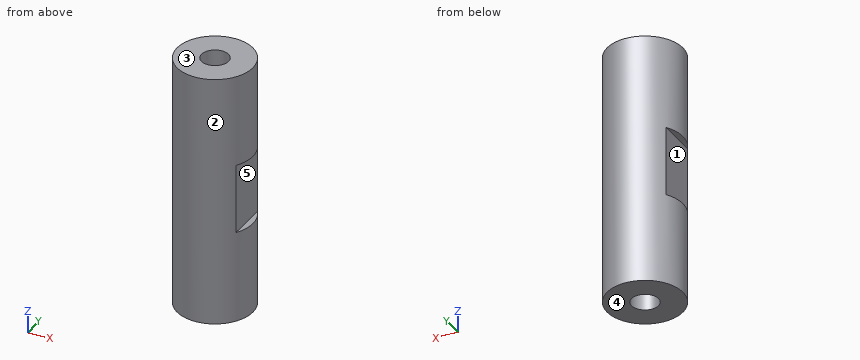
```python
from build123d import *

# Parameters (mm, degrees)
SKETCH_1_R               = 6
SKETCH_1_R_2             = 2.15
EXTRUDE_1_DEPTH          = 40
CUT_EXTRUDE_1_DEPTH      = 41.890096601
CUT_EXTRUDE_1_DEPTH_BACK = 41.890096601
SKETCH_2_W               = 1
SKETCH_2_H               = 11


with BuildPart() as part:
    # Эскиз1 → Бобышка-Вытянуть1 (new body)
    with BuildSketch(Plane.XY):
        Circle(SKETCH_1_R)
        Circle(SKETCH_1_R_2, mode=Mode.SUBTRACT)
    extrude(amount=EXTRUDE_1_DEPTH)

    # Эскиз2 → Вырез-Вытянуть1 (cut, two sides: drawn at the far end of the back side and taken through both)
    with BuildSketch(Plane(origin=(0, 0, 0), x_dir=(1, 0, 0), z_dir=(0, 1, 0)).offset(-CUT_EXTRUDE_1_DEPTH_BACK)):
        with Locations((-5.5, -20)):
            Rectangle(SKETCH_2_W, SKETCH_2_H)
        with Locations((5.5, -20)):
            Rectangle(SKETCH_2_W, SKETCH_2_H)
    extrude(amount=CUT_EXTRUDE_1_DEPTH + CUT_EXTRUDE_1_DEPTH_BACK, mode=Mode.SUBTRACT)


solid = part.part
```
Can you work these out from the model? Positions are in its coordinate system, mm. Face numbers are marked on the shaded views. A direction names the side the tool comes from. Give positions to 0.01 mm unless a question says otherwise; leave off trailing zeros. Loops run counter-clockwise (first coordinate to the right, second up) from the corner with the lowest first, then second, coordinate; pieces in that order, holes last. Notation, with made-up numbers: M 89,61.25 L 145,61.25 A26 ccw 145,98.25 Z; hole C 14.25,46 d4. An arc over 180 degrees is marked long. One line per item, written item: value.
(1) Will these pins go through, and if not, where does the flat tip stop? pin 1 (1 mm diameter, centred on x = 1, z = 6, fed in from +Y); pin 2 (2 mm diameter, centred on x = 3.5, z = 10, fed in from +Y); pin 3 (6 mm diameter, centred on y = -3.5, z = 28, fed in from -X).
Returned:
pin 1: y = 5.98
pin 2: y = 5.45
pin 3: x = -5.98
(2) We'd pull the mould along Z, two halves only. Please class the marked faces 3, 4 and 5: released by +Z, released by -Z, zero draft, split by the parting line, or undercut.
Returned:
face 3: released by +Z
face 4: released by -Z
face 5: undercut
(3) I need wall thicknesses on line 1 (Y direction, x = 0, z = 28); line 2 (X direction, y = 3.25, z = 22); line 3 (Z direction, x = 5.75, y = -1.25). Which ranges of each line are inside material? Lowest first, please.
Returned:
line 1: -6 to -2.15, 2.15 to 6
line 2: -5 to 5
line 3: 0 to 14.5, 25.5 to 40
(4) Suppose I cut it at B-B on y = 0. List the corners of the cut face in (x, z) for me, plus the area to 3 significant figures.
Returned:
outline: M -6,0 L -2.15,0 L -2.15,40 L -6,40 L -6,25.5 L -5,25.5 L -5,14.5 L -6,14.5 Z; M 2.15,0 L 6,0 L 6,14.5 L 5,14.5 L 5,25.5 L 6,25.5 L 6,40 L 2.15,40 Z
area: 286 mm^2
(5) Suppose I cut it at C-C on z = 26. List the corners of the cut face in (x, y) for me, plus the area to 3 significant figures.
Returned:
outline: C 0,0 d12; hole C 0,0 d4.3
area: 98.6 mm^2
(6) Suppose I cut it at A-A on x = 0. List the corners of the cut face in (y, z) for me.
Returned:
outline: M -6,0 L -2.15,0 L -2.15,40 L -6,40 Z; M 2.15,0 L 6,0 L 6,40 L 2.15,40 Z
(7) Suppose I cut it at D-D on y = 2.75. List the corners of the cut face in (x, z) for me, plus the area to 3 significant figures.
Returned:
outline: M -5.33,0 L 5.33,0 L 5.33,14.5 L 5,14.5 L 5,25.5 L 5.33,25.5 L 5.33,40 L -5.33,40 L -5.33,25.5 L -5,25.5 L -5,14.5 L -5.33,14.5 Z
area: 419 mm^2
(8) Which directions (+Z, -Z, +X, -X, +Y, -Y) give clear straight access to the entire face, cutting with the end or side of a thin tool? Please do the marked faces 1 and 2.
Returned:
face 1: -X, +Y, -Y
face 2: +Z, -Z
